from build123d import *

# Parameters (mm, degrees)
F0_R     = 375.9060987096
F1_DEPTH = 270.80607
F2_R     = 149.3370096155
F3_DEPTH = 705.40455
F4_R     = 4.7459118068
F4_R_2   = 59.6341764552
F5_DEPTH = 465.10949
F7_DEPTH = 25.4


with BuildPart() as f1:
    # F0 (on Front) → F1 (new body)
    with BuildSketch(Plane.XZ):
        Circle(F0_R)
    extrude(amount=F1_DEPTH)

    # F2 (on Front) → F3 (cut)
    with BuildSketch(Plane.XZ):
        Circle(F2_R)
    extrude(amount=F3_DEPTH, mode=Mode.SUBTRACT)

    # F4 (on Front) → F5 (join)
    with BuildSketch(Plane.XZ):
        with Locations((0, 272.8897631168)):
            Circle(F4_R)
        with Locations((36.3853052258, 212.7749174833)):
            Circle(F4_R_2)
    extrude(amount=F5_DEPTH)

    # F7 (add): a face of the model
    f7_faces = [f1.faces().sort_by_distance(p)[0] for p in [
        (-365.2738686502, 0, 0),
    ]]
    extrude(f7_faces, amount=F7_DEPTH)


solid = f1.part
For this review, take the finished solid that the model builds, in its own axes (mm). A direction names the side the tool comes from. Give positions to 0.01 mm unless a question says otherwise; leave off trailing zeros. Order: outer loops, then holes, each group sorted by start corner. A loop starts at its lowest first (then second) coordinate and runs counter-clockwise, first axis right, second up. Notation, with made-up numbers: M 19,0 L 24,0 A13 cw 24,15 Z; hole C -29.5,11 d5. An arc over 180 degrees is marked long. Answer in a Markdown table with one row per item. Add a question column.
(1) Consider section A-A on z = 0. State the section outline as (x, y) points.
(2) Consider section C-C on y = -209. State the section outline as (x, z) points, and give its area (3 significant figures).
(3) Consider section D-D on z = 242. State the section outline as (x, y) points, and give its area (3 significant figures).
(4) Mouldability with a two-part tool opening along X and no side actions: class faces 1 (the face through (-19.441, -124.776, 148.066)), 2 (the face through (-5, 25.4, -162)), 3 (the face through (-298.31, -124.78, -228.73)) as +X half, -X half, draft (parallel to the pull), parting line (faces both ways), or undercut.
(5) Wall thickness on probe 1 along Z at (x, y) = (0, -93.5); probe 2 along X at (y, z) = (-222.5, -106); probe 3 along Y at (x, z) = (191, -92): over which ranges is each line inside the solid? List them lowest first. Write a range as [from, to].
(6) For faces 4 (the face through (63.903, -366.598, 159.869)), 5 (the face through (36, -465.109, 214)), list the 3-axis set-ups (+Z, -Z, +X, -X, +Y, -Y) from which the entire face can be reached by the end or side of a thin tool; tool diameter is ignored.
(7) Consider section B-B on x = -103. State the section outline as (y, z) points, and give its area (3 significant figures).
(8) For pin 1 (1.5 mm diameter, centred on x = -142, z = -259.5, fed in from -Y); pin 2 (1 mm diameter, centred on x = 173, y = -39, fed in from -Z); pin 3 (6 mm diameter, centred on x = -18.5, y = -345.5, fed in from +Z), all flat-tipped, find the tip position at first contact; note any pin that passes through.
Evaluation:
| question | item | result |
|---|---|---|
| 1 | outline | M -375.91,-270.81 L -149.34,-270.81 L -149.34,25.4 L -375.91,25.4 Z; M 149.34,-270.81 L 375.91,-270.81 L 375.91,25.4 L 149.34,25.4 Z |
| 2 | outline | C 0,0 d751.81; hole C 0,0 d298.67 |
| 2 | area | 374,000 mm^2 |
| 3 | outline | M -287.65,-270.81 L -15.6,-270.81 L -15.6,-465.11 L 88.37,-465.11 L 88.37,-270.81 L 287.65,-270.81 L 287.65,25.4 L -287.65,25.4 Z |
| 3 | area | 191,000 mm^2 |
| 4 | face 1 | undercut |
| 4 | face 2 | draft |
| 4 | face 3 | parting line |
| 5 | probe 1 | z = [-375.91, -149.34], [149.34, 375.91] |
| 5 | probe 2 | x = [-360.65, -105.19], [105.19, 360.65] |
| 5 | probe 3 | y = [-270.81, 25.4] |
| 6 | face 4 | -Y |
| 6 | face 5 | +Z, -Z, +X, -X, -Y |
| 7 | outline | M -270.81,-361.52 L 25.4,-361.52 L 25.4,-108.13 L -270.81,-108.13 Z; M -270.81,108.13 L 25.4,108.13 L 25.4,361.52 L -270.81,361.52 Z |
| 7 | area | 150,000 mm^2 |
| 8 | pin 1 | stops at y = -270.81 |
| 8 | pin 2 | stops at z = -333.99 |
| 8 | pin 3 | stops at z = 242.17 |
